Could you check a few things on this model? Use its own coordinates, in mm. Face numbers are marked on the shaded views. Give positions to 0.01 mm unless a question says otherwise; leave off trailing zeros. Write each loop counter-clockwise with the first axis right and the second up, starting at its lowest first coordinate (ties: lowest second). Pieces come first, ordered by that corner, then holes. Notation, with made-up numbers: M -36.75,24.5 L -3.75,24.5 A27 cw -3.75,60.5 Z; hole C 78,87.5 d11. An arc over 180 degrees is marked long. One line per item, written item: value.
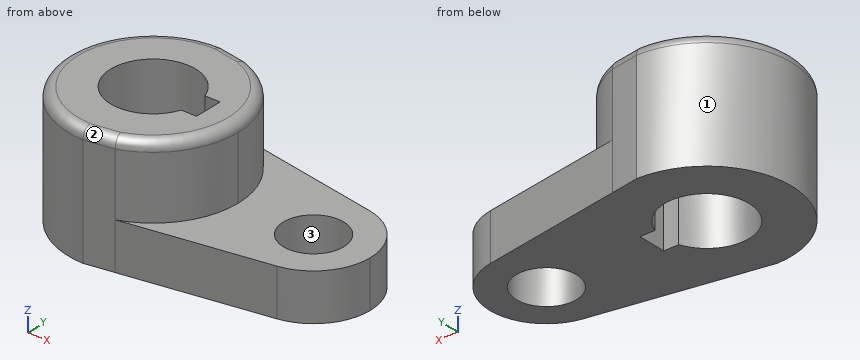
```python
from build123d import *

# Parameters (mm, degrees)
F1_DEPTH    = 40.2336
F0_R        = 10.16
F2_DEPTH    = 15.7734
F3_T1_DEPTH = 37.7177817865
F3_T3_DEPTH = 37.7177817865
F3_T6_ANGLE = 213.1574660215
F3_T8_ANGLE = 174.2489977384


# Not quite as in the source:
# - a fillet or chamfer that OpenCascade refuses, or shapes differently, is made with other operations: its cross-section is extruded or revolved along the edge and cut away or added


with BuildPart() as f1:
    # F0 (on Top) → F1 (new body)
    with BuildSketch(Plane.XY):
        with BuildLine():
            Line((-19.1519816242, 26.9452959039), (-28.6641661078, 28.575))
            ThreePointArc((-28.6641661078, 28.575), (-57.2391661078, 0), (-28.6641661078, -28.575))
            Line((-28.6641661078, -28.575), (-19.1519816242, -26.9452959039))
            ThreePointArc((-19.1519816242, -26.9452959039), (-5.3367005723, -16.5033322905), (-0.0891661078, 0))
            ThreePointArc((-0.0891661078, 0), (-5.3367005723, 16.5033322905), (-19.1519816242, 26.9452959039))
        make_face()
        with BuildLine():
            ThreePointArc((-15.2164012284, -4.826), (-42.9516661078, 0), (-15.2164012284, 4.826))
            Line((-15.2164012284, 4.826), (-10.1348661078, 4.826))
            Line((-10.1348661078, 4.826), (-10.1348661078, -4.826))
            Line((-10.1348661078, -4.826), (-15.2164012284, -4.826))
        make_face(mode=Mode.SUBTRACT)
    extrude(amount=F1_DEPTH)

    # F0 (on Top) → F2 (join)
    with BuildSketch(Plane.XY):
        with BuildLine():
            Line((28.5277611544, 18.7764181619), (-19.1519816242, 26.9452959039))
            ThreePointArc((-19.1519816242, 26.9452959039), (-5.3367005723, 16.5033322905), (-0.0891661078, 0))
            ThreePointArc((-0.0891661078, 0), (-5.3367005723, -16.5033322905), (-19.1519816242, -26.9452959039))
            Line((-19.1519816242, -26.9452959039), (28.5277611544, -18.7764181619))
            ThreePointArc((28.5277611544, -18.7764181619), (6.2608338922, 0), (28.5277611544, 18.7764181619))
        make_face()
        with BuildLine():
            ThreePointArc((44.3608338922, 0), (39.8742291753, 12.2804730295), (28.5277611544, 18.7764181619))
            ThreePointArc((28.5277611544, 18.7764181619), (6.2608338922, 0), (28.5277611544, -18.7764181619))
            ThreePointArc((28.5277611544, -18.7764181619), (39.8742291753, -12.2804730295), (44.3608338922, 0))
        make_face()
        with Locations((25.3108338922, 0)):
            Circle(F0_R, mode=Mode.SUBTRACT)
    extrude(amount=F2_DEPTH)

    # F3: fillet of radius 3.302 on 4 edges, made by hand

    # F3_s2 → F3_t1 (cut)
    with BuildSketch(Plane(origin=(-46.4348249971, -7.955588396, 0), x_dir=(0, 0, 1), z_dir=(0.9856387487, 0.1688675728, 0))):
        with BuildLine():
            ThreePointArc((36.9316, 23.3241790854), (39.2664665915, 22.3570456768), (40.2336, 20.0221790854))
            Line((40.2336, 20.0221790854), (40.2336, 23.3241790854))
            Line((40.2336, 23.3241790854), (36.9316, 23.3241790854))
        make_face()
    extrude(amount=F3_T1_DEPTH, mode=Mode.SUBTRACT)

    # F3_s4 → F3_t3 (cut)
    with BuildSketch(Plane(origin=(-9.258717755, 1.5862781337, 0), x_dir=(0, 0, 1), z_dir=(-0.9856387487, 0.1688675728, 0))):
        with BuildLine():
            ThreePointArc((36.9316, 23.3241790854), (39.2664665915, 22.3570456768), (40.2336, 20.0221790854))
            Line((40.2336, 20.0221790854), (40.2336, 23.3241790854))
            Line((40.2336, 23.3241790854), (36.9316, 23.3241790854))
        make_face()
    extrude(amount=F3_T3_DEPTH, mode=Mode.SUBTRACT)

    # F3_s5 → F3_t6 (revolve, cut)
    with BuildSketch(Plane(origin=(-26.3304812045, 7.8388166507, 0), x_dir=(0, 0, 1), z_dir=(0.95842855, -0.2853326385, 0))):
        with BuildLine():
            ThreePointArc((36.9316, -20.3961778531), (39.2664665915, -19.4290444446), (40.2336, -17.0941778531))
            Line((40.2336, -17.0941778531), (40.2336, -20.3961778531))
            Line((40.2336, -20.3961778531), (36.9316, -20.3961778531))
        make_face()
    revolve(axis=Axis((-28.6641661078, 0, 40.2336), (0, 0, 1)), revolution_arc=F3_T6_ANGLE, mode=Mode.SUBTRACT)

    # F3_s7 → F3_t8 (revolve, cut)
    with BuildSketch(Plane(origin=(-28.5920293734, 1.4361530661, 0), x_dir=(0, 0, 1), z_dir=(-0.9987408987, 0.0501658971, 0))):
        with BuildLine():
            ThreePointArc((40.2336, 23.835036392), (39.2664665915, 26.1699029835), (36.9316, 27.137036392))
            Line((36.9316, 27.137036392), (40.2336, 27.137036392))
            Line((40.2336, 27.137036392), (40.2336, 23.835036392))
        make_face()
    revolve(axis=Axis((-28.6641661078, 0, 40.2336), (0, 0, -1)), revolution_arc=F3_T8_ANGLE, mode=Mode.SUBTRACT)


solid = f1.part
```
1) If we section it at B-B, the plane y = -2.5: Give the number of separate pieces and of enclosed holes in the cut face, then the cut area to 3 significant figures.
Outcome:
separate pieces: 3
enclosed holes: 0
area: 1,360 mm^2
2) I'm going to push flat-ended pins straight in: pin 1 (1 mm diameter, centred on y = -22.5, z = 36, fed in from -X); pin 2 (7.5 mm diameter, centred on y = 1, z = 25.5, fed in from -X); pin 3 (2 mm diameter, centred on x = 33, z = 12.5, fed in from -Y). Where does each tip first touch, or does it pass through?
Outcome:
pin 1: stops at x = -46.9
pin 2: stops at x = -57.24
pin 3: stops at y = -17.84
3) We'd pull the mould along Y, two halves only. Please class the marked faces 1, 2 and 3: pulls with the +Y half, pulls with the -Y half, needs draft (parallel to the pull), parting line crosses it, or undercut.
Outcome:
face 1: parting line crosses it
face 2: pulls with the -Y half
face 3: undercut
4) Please list where these lines run through material, in increasing order: L1, parallel to X at y = 0, z = 32.5; L2, parallel to Z at x = -5.5, y = 11; L3, parallel to Z at x = 19, y = 18.5. Write a range as from..to.
Outcome:
L1: x = -57.24..-42.95, -10.13..-0.09
L2: z = 0..40.21
L3: z = 0..15.77
5) If we section it at C-C, the plane x = 13: Write out the boundary of the cut face in (y, z), then the cut area to 3 significant figures.
Outcome:
outline: M -21.44,0 L 21.44,0 L 21.44,15.77 L -21.44,15.77 Z
area: 676 mm^2
